Verification items for the finished model (mm, model axes). A direction names the side the tool comes from. Coordinates: 2 decimals unless noted, no trailing zeros. Return JSON: item names as keys, results as strings. Group by question number.
1. Material ranges on line 1 along X through (y, z) = (31, 34); line 2 along X through (y, z) = (-28, 30); line 3 along Y through (x, z) = (-30.5, 13), recorded low to high.
2. Mould release check, pull along Y, two halves, no side actions. Record for faces 6 (the conical face through (23.746, 28.166, 11.309)), 7 (the cylindrical face through (-13.279, 33.862, 9.396)), 8 (the conical face through (20.392, 20.726, 57.276)): +Y half, -Y half, draft (parallel to the pull), parting line (faces both ways), or undercut.
3. Gauge pin test, flat ends, axial feed: pin 1 (12 mm diameter, centred on x = -20.4, y = 22.21, fed in from +Z); pin 2 (9 mm diameter, centred on x = 24.95, z = 11.81, fed in from +Y); pin 3 (17 mm diameter, centred on x = -22.28, y = 22.98, fed in from +Z); pin 4 (12 mm diameter, centred on y = 3.62, z = 30.03, fed in from +X). Record the tip position at first contact, or that the pin passes through.
4. Set-up check for faces 1 (the cylindrical face through (-27.33, 19.34, 62.97)), 2 (the cylindrical face through (-34.277, -18.232, 53.679)), 3 (the conical face through (-2.435, -28.166, 28.46)), 4 (the cylindrical face through (16.85, 33.86, 32.51)), 5 (the cylindrical face through (7.493, -0.33, 2.028)): record each of +Z, -Z, +X, -X, +Y, -Y from which the full face is reachable in a straight line by a thin tool's end or side.
```python
from build123d import *

# Parameters (mm, degrees)
F0_W      = 72.6099312305
F0_H      = 71.7801898718
F1_DEPTH  = 65
F3_D      = 15
F3_DEPTH  = 4
F3_TIP    = 4.5064546427
F6_D      = 15
F6_DEPTH  = 4
F6_TIP    = 4.5064546427
F7_D      = 15
F7_DEPTH  = 4
F7_TIP    = 4.5064546427
F12_D     = 15
F12_DEPTH = 4
F12_TIP   = 4.5064546427
F13_D     = 15
F13_DEPTH = 4
F13_TIP   = 4.5064546427
F14_D     = 15
F14_DEPTH = 4
F14_TIP   = 4.5064546427
F15_D     = 15
F15_DEPTH = 4
F15_TIP   = 4.5064546427
F22_D     = 15
F22_DEPTH = 4
F22_TIP   = 4.5064546427
F23_D     = 15
F23_DEPTH = 4
F23_TIP   = 4.5064546427
F24_D     = 15
F24_DEPTH = 4
F24_TIP   = 4.5064546427
F25_D     = 15
F25_DEPTH = 4
F25_TIP   = 4.5064546427
F26_D     = 15
F26_DEPTH = 4
F26_TIP   = 4.5064546427
F27_D     = 15
F27_DEPTH = 4
F27_TIP   = 4.5064546427
F31_D     = 15
F31_DEPTH = 4
F31_TIP   = 4.5064546427
F32_D     = 15
F32_DEPTH = 4
F32_TIP   = 4.5064546427
F33_D     = 15
F33_DEPTH = 4
F33_TIP   = 4.5064546427
F37_D     = 15
F37_DEPTH = 4
F37_TIP   = 4.5064546427
F38_D     = 15
F38_DEPTH = 4
F38_TIP   = 4.5064546427
F41_D     = 15
F41_DEPTH = 4
F41_TIP   = 4.5064546427
F42_D     = 15
F42_DEPTH = 4
F42_TIP   = 4.5064546427
F43_D     = 15
F43_DEPTH = 4
F43_TIP   = 4.5064546427


with BuildPart() as f1:
    # F0 (on Top) → F1 (new body)
    with BuildSketch(Plane.XY):
        Rectangle(F0_W, F0_H)
    extrude(amount=F1_DEPTH)

    # F3
    with Locations(Plane.XZ.offset(35.8900949359)):
        with Locations((-2.1530347876, 29.7311879694)):
            Hole(F3_D / 2, depth=F3_DEPTH)
            with Locations((0, 0, -(F3_DEPTH + F3_TIP / 2))):  # 118° drill point
                Cone(0, F3_D / 2, F3_TIP, mode=Mode.SUBTRACT)

    # F6
    with Locations(Plane(origin=(-36.3049656153, 0, 0), x_dir=(0, -1, 0), z_dir=(-1, 0, 0))):
        with Locations((22.2641993314, 47.3547130823)):
            Hole(F6_D / 2, depth=F6_DEPTH)
            with Locations((0, 0, -(F6_DEPTH + F6_TIP / 2))):  # 118° drill point
                Cone(0, F6_D / 2, F6_TIP, mode=Mode.SUBTRACT)

    # F7
    with Locations(Plane(origin=(-36.3049656153, 0, 0), x_dir=(0, -1, 0), z_dir=(-1, 0, 0))):
        with Locations((-25.2181496471, 10.9740728512)):
            Hole(F7_D / 2, depth=F7_DEPTH)
            with Locations((0, 0, -(F7_DEPTH + F7_TIP / 2))):  # 118° drill point
                Cone(0, F7_D / 2, F7_TIP, mode=Mode.SUBTRACT)

    # F12
    with Locations(Plane.XY.offset(65)):
        with Locations((-20.3992947936, 22.2076252103)):
            Hole(F12_D / 2, depth=F12_DEPTH)
            with Locations((0, 0, -(F12_DEPTH + F12_TIP / 2))):  # 118° drill point
                Cone(0, F12_D / 2, F12_TIP, mode=Mode.SUBTRACT)

    # F13
    with Locations(Plane.XY.offset(65)):
        with Locations((21.4252322912, 21.5187519789)):
            Hole(F13_D / 2, depth=F13_DEPTH)
            with Locations((0, 0, -(F13_DEPTH + F13_TIP / 2))):  # 118° drill point
                Cone(0, F13_D / 2, F13_TIP, mode=Mode.SUBTRACT)

    # F14
    with Locations(Plane.XY.offset(65)):
        with Locations((-21.5802267194, -23.0612829328)):
            Hole(F14_D / 2, depth=F14_DEPTH)
            with Locations((0, 0, -(F14_DEPTH + F14_TIP / 2))):  # 118° drill point
                Cone(0, F14_D / 2, F14_TIP, mode=Mode.SUBTRACT)

    # F15
    with Locations(Plane.XY.offset(65)):
        with Locations((22.606164217, -22.4708169699)):
            Hole(F15_D / 2, depth=F15_DEPTH)
            with Locations((0, 0, -(F15_DEPTH + F15_TIP / 2))):  # 118° drill point
                Cone(0, F15_D / 2, F15_TIP, mode=Mode.SUBTRACT)

    # F22
    with Locations(Plane(origin=(0, 35.8900949359, 0), x_dir=(-1, 0, 0), z_dir=(0, 1, 0))):
        with Locations((-23.0850540102, 50.5671985447)):
            Hole(F22_D / 2, depth=F22_DEPTH)
            with Locations((0, 0, -(F22_DEPTH + F22_TIP / 2))):  # 118° drill point
                Cone(0, F22_D / 2, F22_TIP, mode=Mode.SUBTRACT)

    # F23
    with Locations(Plane(origin=(0, 35.8900949359, 0), x_dir=(-1, 0, 0), z_dir=(0, 1, 0))):
        with Locations((-24.3417993188, 32.1762934327)):
            Hole(F23_D / 2, depth=F23_DEPTH)
            with Locations((0, 0, -(F23_DEPTH + F23_TIP / 2))):  # 118° drill point
                Cone(0, F23_D / 2, F23_TIP, mode=Mode.SUBTRACT)

    # F24
    with Locations(Plane(origin=(0, 35.8900949359, 0), x_dir=(-1, 0, 0), z_dir=(0, 1, 0))):
        with Locations((-24.9489825219, 11.8078188971)):
            Hole(F24_D / 2, depth=F24_DEPTH)
            with Locations((0, 0, -(F24_DEPTH + F24_TIP / 2))):  # 118° drill point
                Cone(0, F24_D / 2, F24_TIP, mode=Mode.SUBTRACT)

    # F25
    with Locations(Plane(origin=(0, 35.8900949359, 0), x_dir=(-1, 0, 0), z_dir=(0, 1, 0))):
        with Locations((22.4829968065, 50.1865930855)):
            Hole(F25_D / 2, depth=F25_DEPTH)
            with Locations((0, 0, -(F25_DEPTH + F25_TIP / 2))):  # 118° drill point
                Cone(0, F25_D / 2, F25_TIP, mode=Mode.SUBTRACT)

    # F26
    with Locations(Plane(origin=(0, 35.8900949359, 0), x_dir=(-1, 0, 0), z_dir=(0, 1, 0))):
        with Locations((21.5991660953, 31.6905751824)):
            Hole(F26_D / 2, depth=F26_DEPTH)
            with Locations((0, 0, -(F26_DEPTH + F26_TIP / 2))):  # 118° drill point
                Cone(0, F26_D / 2, F26_TIP, mode=Mode.SUBTRACT)

    # F27
    with Locations(Plane(origin=(0, 35.8900949359, 0), x_dir=(-1, 0, 0), z_dir=(0, 1, 0))):
        with Locations((20.2071741223, 12.2690275311)):
            Hole(F27_D / 2, depth=F27_DEPTH)
            with Locations((0, 0, -(F27_DEPTH + F27_TIP / 2))):  # 118° drill point
                Cone(0, F27_D / 2, F27_TIP, mode=Mode.SUBTRACT)

    # F31
    with Locations(Plane.YZ.offset(36.3049656153)):
        with Locations((24.3696309626, 49.1544306278)):
            Hole(F31_D / 2, depth=F31_DEPTH)
            with Locations((0, 0, -(F31_DEPTH + F31_TIP / 2))):  # 118° drill point
                Cone(0, F31_D / 2, F31_TIP, mode=Mode.SUBTRACT)

    # F32
    with Locations(Plane.YZ.offset(36.3049656153)):
        with Locations((3.6195591092, 30.0324633718)):
            Hole(F32_D / 2, depth=F32_DEPTH)
            with Locations((0, 0, -(F32_DEPTH + F32_TIP / 2))):  # 118° drill point
                Cone(0, F32_D / 2, F32_TIP, mode=Mode.SUBTRACT)

    # F33
    with Locations(Plane.YZ.offset(36.3049656153)):
        with Locations((-24.0738447756, 11.9759794325)):
            Hole(F33_D / 2, depth=F33_DEPTH)
            with Locations((0, 0, -(F33_DEPTH + F33_TIP / 2))):  # 118° drill point
                Cone(0, F33_D / 2, F33_TIP, mode=Mode.SUBTRACT)

    # F37
    with Locations(Plane(origin=(0, 0, 0), x_dir=(1, 0, 0), z_dir=(0, 0, -1))):
        with Locations((-24.6889404953, 23.873642087)):
            Hole(F37_D / 2, depth=F37_DEPTH)
            with Locations((0, 0, -(F37_DEPTH + F37_TIP / 2))):  # 118° drill point
                Cone(0, F37_D / 2, F37_TIP, mode=Mode.SUBTRACT)

    # F38
    with Locations(Plane(origin=(0, 0, 0), x_dir=(1, 0, 0), z_dir=(0, 0, -1))):
        with Locations((0, 0)):
            Hole(F38_D / 2, depth=F38_DEPTH)
            with Locations((0, 0, -(F38_DEPTH + F38_TIP / 2))):  # 118° drill point
                Cone(0, F38_D / 2, F38_TIP, mode=Mode.SUBTRACT)

    # F41
    with Locations(Plane(origin=(0, 0, 0), x_dir=(1, 0, 0), z_dir=(0, 0, -1))):
        with Locations((25.4348441958, 25.4543684423)):
            Hole(F41_D / 2, depth=F41_DEPTH)
            with Locations((0, 0, -(F41_DEPTH + F41_TIP / 2))):  # 118° drill point
                Cone(0, F41_D / 2, F41_TIP, mode=Mode.SUBTRACT)

    # F42
    with Locations(Plane(origin=(0, 0, 0), x_dir=(1, 0, 0), z_dir=(0, 0, -1))):
        with Locations((-22.2828052938, -22.9848101735)):
            Hole(F42_D / 2, depth=F42_DEPTH)
            with Locations((0, 0, -(F42_DEPTH + F42_TIP / 2))):  # 118° drill point
                Cone(0, F42_D / 2, F42_TIP, mode=Mode.SUBTRACT)

    # F43
    with Locations(Plane(origin=(0, 0, 0), x_dir=(1, 0, 0), z_dir=(0, 0, -1))):
        with Locations((21.6378718615, -21.6745659709)):
            Hole(F43_D / 2, depth=F43_DEPTH)
            with Locations((0, 0, -(F43_DEPTH + F43_TIP / 2))):  # 118° drill point
                Cone(0, F43_D / 2, F43_TIP, mode=Mode.SUBTRACT)


solid = f1.part
```
Answers follow:
{
 "1": {"line 1": "-36.3 to -27.16, -16.04 to 18.61, 30.08 to 36.3", "line 2": "-36.3 to -3.14, -1.16 to 36.3", "line 3": "-35.89 to 21.2, 29.23 to 35.89"},
 "2": {"face 6": "+Y half", "face 7": "draft", "face 8": "undercut"},
 "3": {"pin 1": "z = 60.1", "pin 2": "y = 30.09", "pin 3": "z = 65", "pin 4": "x = 31.41"},
 "4": {"face 1": "+Z", "face 2": "-X", "face 3": "-Y", "face 4": "+Y", "face 5": "-Z"}
}
